from build123d import *

# Parameters (mm, degrees)
SKETCH1_W           = 36.83
SKETCH1_H           = 5.529791667
SKETCH5_R           = 27.5
BOSS_EXTRUDE1_DEPTH = 0.001
SKETCH19_R          = 12.7
CUT_EXTRUDE6_DEPTH  = 6.530791667
CIRPATTERN1_COUNT   = 4
CUT_EXTRUDE7_DEPTH  = 6.529791667
CIRPATTERN2_COUNT   = 4
CHAMFER1_SIZE       = 3.175
SKETCH28_R          = 16.2052
SKETCH28_R_2        = 13.97
CUT_EXTRUDE17_DEPTH = 1.3208


with BuildPart() as part:
    # Sketch1 → Revolve1 (revolve)
    with BuildSketch(Plane(origin=(0, 0, 0), x_dir=(-1, 0, 0), z_dir=(0, 0, -1))):
        with Locations((-18.415, -2.764895834)):
            Rectangle(SKETCH1_W, SKETCH1_H)
    revolve(axis=Axis((0, -5.529791667, 0), (0, 1, 0)))

    # Sketch5 → Boss-Extrude1 (add)
    with BuildSketch(Plane.XZ.offset(5.529791667)):
        Circle(SKETCH5_R)
    extrude(amount=BOSS_EXTRUDE1_DEPTH)

    # Sketch12 → #4-40 Tapped Hole1 (revolve, cut)
    with BuildSketch(Plane(origin=(-14.601755032, -5.530791667, 14.601755032), x_dir=(0, 0, -1), z_dir=(1, 0, 0))):
        Polygon((0, 0), (0, 3.981152758), (1.1303, 3.302), (1.1303, 0), align=None)
    f_4_40_tapped_hole1 = revolve(axis=Axis((-14.601755032, -11.880791667, 14.601755032), (0, 1, 0)), mode=Mode.SUBTRACT)

    # Sketch19 → Cut-Extrude6 (cut, through all)
    with BuildSketch(Plane.XZ.offset(5.530791667)):
        Circle(SKETCH19_R)
    extrude(amount=-CUT_EXTRUDE6_DEPTH, mode=Mode.SUBTRACT)

    # CirPattern1: #4-40 Tapped Hole1 ×4 about axis
    cirpattern1_axis = Axis((0, 0, 0), (0, 1, 0))
    for i in range(1, CIRPATTERN1_COUNT):
        add(f_4_40_tapped_hole1.rotate(cirpattern1_axis, i * 360 / CIRPATTERN1_COUNT), mode=Mode.SUBTRACT)

    # Sketch20 → Cut-Extrude7 (cut, through all)
    with BuildSketch(Plane(origin=(0, -5.529791667, 0), x_dir=(-1, 0, 0), z_dir=(0, -1, 0))):
        with BuildLine():
            Line((2.5, -32.5), (2.5, -42.5))
            ThreePointArc((2.5, -42.5), (0, -45), (-2.5, -42.5))
            Line((-2.5, -42.5), (-2.5, -32.5))
            ThreePointArc((-2.5, -32.5), (0, -30), (2.5, -32.5))
        make_face()
    cut_extrude7 = extrude(amount=-CUT_EXTRUDE7_DEPTH, mode=Mode.SUBTRACT)

    # CirPattern2: Cut-Extrude7 ×4 about axis
    cirpattern2_axis = Axis((0, 0, 0), (0, 1, 0))
    for i in range(1, CIRPATTERN2_COUNT):
        add(cut_extrude7.rotate(cirpattern2_axis, i * 360 / CIRPATTERN2_COUNT), mode=Mode.SUBTRACT)

    # Chamfer1
    chamfer1_edges = [part.edges().sort_by_distance(p)[0] for p in [
        (-12.7, 0, 0),
    ]]
    chamfer(chamfer1_edges, length=CHAMFER1_SIZE)

    # Sketch28 → Cut-Extrude17 (cut)
    with BuildSketch(Plane.XZ.offset(5.530791667)):
        Circle(SKETCH28_R)
        Circle(SKETCH28_R_2, mode=Mode.SUBTRACT)
    extrude(amount=-CUT_EXTRUDE17_DEPTH, mode=Mode.SUBTRACT)


solid = part.part
Verification items for the finished model (mm, model axes). A direction names the side the tool comes from. Give positions to 0.01 mm unless a question says otherwise; leave off trailing zeros.
1) Draft check along X on faces 1 (the flat face through (2.5, -3, 35)), 2 (the flat face through (-35, -3, -2.5)), 3 (the cylindrical face through (25.78, -2.726, 26.303)). Enter one of: pulls with the +X half, pulls with the -X half, needs draft (parallel to the pull), parting line crosses it, or undercut.
2) Thickness scan on line 1 along Z through (x, y) = (0, -4.7); line 2 along X through (y, z) = (-2.25, -14); line 3 along X through (y, z) = (-4.95, -9.5). Record the ranges inside material, lowest first.
3) Set-up check for faces 4 (the flat face through (-2.5, -3, -35)), 5 (the cylindrical face through (-1.82, -4.88, 13.85)), 6 (the flat face through (35, -3, -2.5)), 7 (the flat face through (-2.5, -3, 35)): record each of +Z, -Z, +X, -X, +Y, -Y from which the full face is reachable in a straight line by a thin tool's end or side.
4) Depth check by flat-ended pin: pin 1 Ø1 at (x, y) = (24, -3.5) entering from -Z; pin 2 Ø1.5 at (x, y) = (-15.5, -1.5) entering from -Z; pin 3 Ø1.5 at (y, z) = (-1, -12) entering from +X. Enter the tip coordinate at first touch or a pass-through.
Answers:
1. face 1: undercut
1. face 2: needs draft
1. face 3: pulls with the +X half
2. line 1: z = -30 to -16.21, -13.97 to -12.7, 12.7 to 13.97, 16.21 to 30
2. line 2: x = -34.07 to -15.56, -13.64 to 13.64, 15.56 to 34.07
2. line 3: x = -35.58 to -13.13, -10.24 to -8.43, 8.43 to 10.24, 13.13 to 35.58
3. face 4: -Z, +Y, -Y
3. face 5: -Y
3. face 6: +X, +Y, -Y
3. face 7: +Z, +Y, -Y
4. pin 1: stops at z = -28.36
4. pin 2: stops at z = -33.75
4. pin 3: stops at x = 35.07
